from build123d import *

# Parameters (mm, degrees)
SKETCH2_R                = 1.2
BOSS_EXTRUDE1_DEPTH      = 2.5
BOSS_EXTRUDE1_DEPTH_BACK = 2.5
SWEEP1_PROFILE_R         = 0.2
SKETCH23_R               = 1.2
SKETCH23_R_2             = 1.15
CUT_EXTRUDE1_DEPTH       = 0.5


with BuildPart() as part:
    # Sketch2 → Boss-Extrude1 (new body, two sides)
    with BuildSketch(Plane(origin=(0, 0, 0), x_dir=(1, 0, 0), z_dir=(0, 1, 0))) as boss_extrude1_sk:
        Circle(SKETCH2_R)
    extrude(amount=BOSS_EXTRUDE1_DEPTH)
    extrude(boss_extrude1_sk.sketch, amount=-BOSS_EXTRUDE1_DEPTH_BACK)

    # Sweep1: sweep along a path in Sketch3
    with BuildLine(Plane(origin=(0, 0, 0), x_dir=(0, 0, -1), z_dir=(1, 0, 0))) as sweep1_path:
        Line((0, 2.5), (0, 2.61))
        ThreePointArc((0, 2.61), (-0.351471863, 3.458528137), (-1.2, 3.81))
        Line((-1.2, 3.81), (-3.2, 3.81))
    # Sweep1 profile (on start of the path) → Sweep1 (sweep)
    with BuildSketch(Plane.ZX.offset(2.5)):
        Circle(SWEEP1_PROFILE_R)
    sweep1 = sweep(path=sweep1_path.line)

    # Mirror1: Sweep1 across plane
    add(sweep1.mirror(Plane.ZX))

    # Sketch23 → Cut-Extrude1 (cut)
    with BuildSketch(Plane.XZ.offset(2.5)):
        Circle(SKETCH23_R)
        Circle(SKETCH23_R_2, mode=Mode.SUBTRACT)
    extrude(amount=-CUT_EXTRUDE1_DEPTH, mode=Mode.SUBTRACT)


solid = part.part
Read the model definition and answer for the solid it produces. Units are mm, in the model's axes. Round coordinates to 2 decimals unless told otherwise and drop trailing zeros. Loops run counter-clockwise (first coordinate to the right, second up) from the corner with the lowest first, then second, coordinate; pieces in that order, holes last.
Q1. Each of these flat-tipped pins is pushed along its axis until it touches: pin 1 (0.7 mm diameter, centred on x = 0, z = 0, fed in from -Y); pin 2 (2 mm diameter, centred on y = 1.5, z = 1.5, fed in from -X). Where does it stop, or does it pass through?
Q2. Section D-D on z = -0.7 is taken. Write down the section's boundary in (x, y).
Q3. Section B-B on z = 2 is taken. Write down the section's boundary in (x, y).
Q4. Consider probe 1 along Z at (x, y) = (0, -1); probe 2 along Y at (x, z) = (-1, -0.45); probe 3 along Y at (x, z) = (-0.1, 0.5). Determine where each line is inside the solid, lowest interval first.
Q5. Section C-C on y = 1 is taken. Write down the section's boundary in (x, z).
Q6. Section A-A on x = 0 is taken. Write down the section's boundary in (y, z).
Output:
1. pin 1: stops at y = -3.72
1. pin 2: stops at x = -1.09
2. outline: (-0.97, -2) - (-0.91, -2) - (-0.91, -2.5) - (0.91, -2.5) - (0.91, -2) - (0.97, -2) - (0.97, 2.5) - (-0.97, 2.5) - close
3. outline: circle Ø0.4 at (0, -3.81); circle Ø0.4 at (0, 3.81)
4. probe 1: z = -1.2 to 1.2
4. probe 2: y = -2.5 to 2.5
4. probe 3: y = -3.79 to -3.36, -2.5 to 2.5, 3.36 to 3.79
5. outline: circle Ø2.4 at (0, 0)
6. outline: (-4.01, 1.2) arc R1.4 ccw to (-2.61, -0.2) - (-2.5, -0.2) - (-2.5, -1.15) - (-2, -1.15) - (-2, -1.2) - (2.5, -1.2) - (2.5, -0.2) - (2.61, -0.2) arc R1.4 ccw to (4.01, 1.2) - (4.01, 3.2) - (3.61, 3.2) - (3.61, 1.2) arc R1 cw to (2.61, 0.2) - (2.5, 0.2) - (2.5, 1.2) - (-2, 1.2) - (-2, 1.15) - (-2.5, 1.15) - (-2.5, 0.2) - (-2.61, 0.2) arc R1 cw to (-3.61, 1.2) - (-3.61, 3.2) - (-4.01, 3.2) - close
